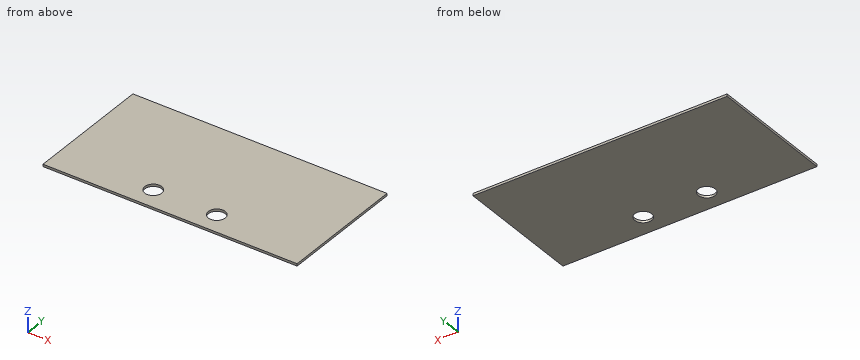
from build123d import *

# Parameters (mm, degrees)
CYLINDER001_R     = 4
CYLINDER001_DEPTH = 1.1
CYLINDER_R        = 4
CYLINDER_DEPTH    = 1.1
BOX_W             = 120
BOX_H             = 60
BOX_DEPTH         = 1.1


with BuildPart() as cylinder001:
    # Cylinder001 → Cylinder001 (new body)
    with BuildSketch(Plane(origin=(75, 10, 0), x_dir=(1, 0, 0), z_dir=(0, 0, 1))):
        Circle(CYLINDER001_R)
    extrude(amount=CYLINDER001_DEPTH)


with BuildPart() as cylinder:
    # Cylinder → Cylinder (new body)
    with BuildSketch(Plane(origin=(45, 10, 0), x_dir=(1, 0, 0), z_dir=(0, 0, 1))):
        Circle(CYLINDER_R)
    extrude(amount=CYLINDER_DEPTH)


with BuildPart() as cut001:
    # Box → Box (new body)
    with BuildSketch(Plane.XY):
        with Locations((60, 30)):
            Rectangle(BOX_W, BOX_H)
    extrude(amount=BOX_DEPTH)

    # Cut: cut Cylinder
    add(cylinder.part, mode=Mode.SUBTRACT)

    # Cut001: cut Cylinder001
    add(cylinder001.part, mode=Mode.SUBTRACT)


solid = cut001.part
Build history of the part. All positions in model axes, mm. Coordinates: 2 decimals unless noted, no trailing zeros. Order: outer loops, then holes, each group sorted by start corner. A loop starts at its lowest first (then second) coordinate and runs counter-clockwise, first axis right, second up. Notation, with made-up numbers: (18, 78) - (56, 78) arc R29 ccw to (56, 113) - close; hole circle Ø6 at (68, 19.25). An arc over 180 degrees is marked (long way). Write each question's results on one line, items separated by ' | '. Start each with the question number.
Item 1: Band-saw the part on A-A on x = 75. Write the cut outline in (y, z).
Item 2: Wall check: probe 1 along Y at (x, z) = (45, 0.6); probe 2 along Y at (x, z) = (46.5, 1). Give the ranges that are in metal, low to high. Write a range as [from, to].
Item 3: Band-saw the part on B-B on y = 10. Write the cut outline in (x, z), and give its area (3 significant figures).
Numbers:
1) outline: (0, 0) - (6, 0) - (6, 1.1) - (0, 1.1) - close; (14, 0) - (60, 0) - (60, 1.1) - (14, 1.1) - close
2) probe 1: [0, 6], [14, 60] | probe 2: [0, 6.29], [13.71, 60]
3) outline: (0, 0) - (41, 0) - (41, 1.1) - (0, 1.1) - close; (49, 0) - (71, 0) - (71, 1.1) - (49, 1.1) - close; (79, 0) - (120, 0) - (120, 1.1) - (79, 1.1) - close | area: 114 mm^2
